Source: CAD feature listing. Evaluate the final solid. Frame: model axes, mm. Face numbers are marked on the shaded views. A direction names the side the tool comes from. Coordinates: 2 decimals unless noted, no trailing zeros. Write each loop counter-clockwise with the first axis right and the second up, starting at its lowest first coordinate (ties: lowest second). Pieces come first, ordered by that corner, then holes. Notation, with made-up numbers: M -7.75,-29 L 25.25,-29 A11 ccw 25.25,-11 Z; hole C 9,-21 d11. An arc over 180 degrees is marked long. One line per item, written item: value. Start each with the question number.
Item 1: Cut plane D-D, the plane x = -25.5. Output: boundary loops of the cut face in (y, z) (3 decimals), then the cut area to 3 significant figures.
Item 2: Set-up query: the marked faces 4 and 5. Return all of +Z, -Z, +X, -X, +Y, -Y with unobstructed straight access to the full face (end or side cutting, diameter ignored); none if empty.
Item 3: Pin query (flat end, axial travel): P1, Ø1.9, axis at y = 0.5, z = 22.5, coming from the -X side; P2, Ø4, axis at x = -18, z = -23.5, coming from the +Y side (3 decimals); P3, Ø5, axis at y = -1, z = 7, coming from the -X side. Return the tip coordinate at first contact, or that it passes through.
Item 4: Cut plane A-A, the plane x = 0. Output: boundary loops of the cut face in (y, z) (3 decimals), then the cut area to 3 significant figures.
Item 5: Ray query, L1, parallel to X at y = -3, z = 6; L2, parallel to X at y = -1.75, z = 15; L3, parallel to Y at x = -23.5, z = -18 (3 decimals). Return the intervals inside material, ascending. Write a range as from..to.
Item 6: Cut plane C-C, the plane y = -0.75. Output: boundary loops of the cut face in (x, z), then the cut area to 3 significant figures.
Item 7: Mould query, pull axis Z, two halves, no side actions, for the marked faces 1, 2 and 3. Classes: released by +Z, released by -Z, zero draft, split by the parting line, or undercut.
Item 8: Cut plane B-B, the plane z = 8. Output: boundary loops of the cut face in (x, y) (3 decimals).
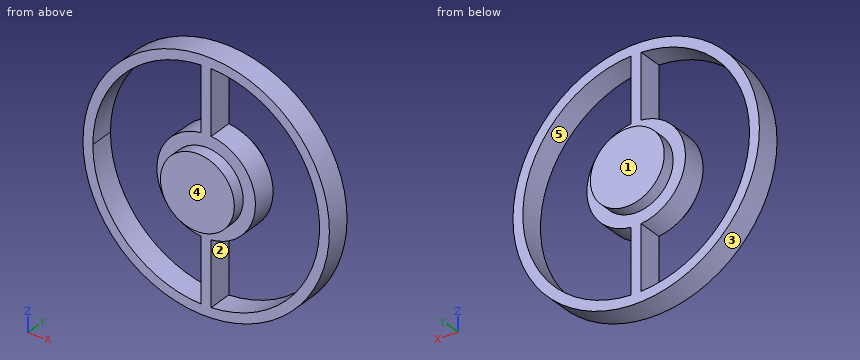
```python
from build123d import *

# Parameters (mm, degrees)
F0_R      = 31.75
F1_DEPTH  = 3.175
F2_R      = 29.21
F3_DEPTH  = 6.351
F4_R      = 12.7
F5_DEPTH  = 3.175
F7_DEPTH  = 3.175
F8_COUNT  = 2
F9_R      = 9.525
F10_DEPTH = 6.35


with BuildPart() as f1:
    # F0 (on Front) → F1 (new body, symmetric)
    with BuildSketch(Plane.XZ):
        Circle(F0_R)
    extrude(amount=F1_DEPTH, both=True)

    # F2 (on face) → F3 (cut, through all)
    with BuildSketch(Plane.XZ.offset(3.175)):
        Circle(F2_R)
    extrude(amount=-F3_DEPTH, mode=Mode.SUBTRACT)



with BuildPart() as f5:
    # F4 (on Front) → F5 (new body, symmetric)
    with BuildSketch(Plane.XZ):
        Circle(F4_R)
    extrude(amount=F5_DEPTH, both=True)


with BuildPart() as f1_1:
    add(f1.part)

    add(f5.part)  # F7 merges F5
    # F6 (on Front) → F7 (join, symmetric)
    with BuildSketch(Plane.XZ):
        Polygon((1.27, 30.9208352119), (0, 30.9208352119), (-1.27, 30.9208352119), (-1.27, 0), (0, 0), (1.27, 0), align=None)
    extrude(amount=F7_DEPTH, both=True)

    # F8: F1 ×2 about axis
    f8_axis = Axis((0, -3.175, 0), (0, 1, 0))


with BuildPart() as f1_2:
    add(f1_1.part)
    for i in range(1, F8_COUNT):
        add(f1_1.part.rotate(f8_axis, i * 360 / F8_COUNT))

    # F9 (on Front) → F10 (join, symmetric)
    with BuildSketch(Plane.XZ):
        Circle(F9_R)
    extrude(amount=F10_DEPTH, both=True)


solid = f1_2.part
```
From the geometry:
1. outline: M -3.175,-18.916 L 3.175,-18.916 L 3.175,-14.247 L -3.175,-14.247 Z; M -3.175,14.247 L 3.175,14.247 L 3.175,18.916 L -3.175,18.916 Z
1. area: 59.3 mm²
2. face 4: +Z, -Z, +X, -X, -Y
2. face 5: +Y, -Y
3. P1: stops at x = -23.32
3. P2: stops at y = 3.175
3. P3: stops at x = -31.43
4. outline: M -6.35,-9.525 L -3.175,-9.525 L -3.175,-31.75 L 3.175,-31.75 L 3.175,-9.525 L 6.35,-9.525 L 6.35,9.525 L 3.175,9.525 L 3.175,31.75 L -3.175,31.75 L -3.175,9.525 L -6.35,9.525 Z
4. area: 524 mm²
5. L1: x = -31.18..-28.59, -11.19..11.19, 28.59..31.18
5. L2: x = -27.98..-25.06, -1.27..1.27, 25.06..27.98
5. L3: y = -3.175..3.175
6. outline: C 0,0 d63.5; hole M -1.27,-29.18 L -1.27,-12.64 A12.7 cw -1.27,12.64 L -1.27,29.18 A29.21 ccw Z; hole M 1.27,-29.18 A29.21 ccw 1.27,29.18 L 1.27,12.64 A12.7 cw 1.27,-12.64 Z
6. area: 1,080 mm²
7. face 1: zero draft
7. face 2: undercut
7. face 3: split by the parting line
8. outline: M -30.726,-3.175 L -28.093,-3.175 L -28.093,3.175 L -30.726,3.175 Z; M -9.864,-3.175 L -5.17,-3.175 L -5.17,-6.35 L 5.17,-6.35 L 5.17,-3.175 L 9.864,-3.175 L 9.864,3.175 L 5.17,3.175 L 5.17,6.35 L -5.17,6.35 L -5.17,3.175 L -9.864,3.175 Z; M 28.093,-3.175 L 30.726,-3.175 L 30.726,3.175 L 28.093,3.175 Z
